The model under review builds one solid part; all positions refer to its coordinate system, in mm. Round coordinates to 2 decimals unless told otherwise and drop trailing zeros. Loops run counter-clockwise (first coordinate to the right, second up) from the corner with the lowest first, then second, coordinate; pieces in that order, holes last. Notation, with made-up numbers: (1, 28.25) -> (27, 28.25) arc R26 cw to (27, 63.25) -> close; hole circle Ø10 at (49, -3). An arc over 180 degrees is marked (long way). Return JSON: item names as keys, results as strings. Group by question number.
```python
from build123d import *

# Parameters (mm, degrees)
SKETCH1_W           = 25.4
SKETCH1_H           = 25.4
SKETCH1_W_2         = 19.05
SKETCH1_H_2         = 19.05
BOSS_EXTRUDE1_DEPTH = 266.7
CUT_EXTRUDE1_REACH  = 271.108
SKETCH3_R           = 6.35
CUT_EXTRUDE2_DEPTH  = 270.108175275


with BuildPart() as part:
    # Sketch1 → Boss-Extrude1 (new body)
    with BuildSketch(Plane.XY):
        with Locations((12.7, 12.7)):
            Rectangle(SKETCH1_W, SKETCH1_H)
        with Locations((12.7, 12.7)):
            Rectangle(SKETCH1_W_2, SKETCH1_H_2, mode=Mode.SUBTRACT)
    extrude(amount=BOSS_EXTRUDE1_DEPTH)

    # Sketch2 → Cut-Extrude1 (cut, up to next)
    with BuildSketch(Plane(origin=(0, 25.4, 0), x_dir=(1, 0, 0), z_dir=(0, 1, 0)), mode=Mode.PRIVATE) as cut_extrude1_sk1:
        Polygon((25.4, -35.938150335), (0, 0), (25.4, 0), align=None)
    cut_extrude1_tool1 = extrude(cut_extrude1_sk1.sketch, amount=-CUT_EXTRUDE1_REACH, mode=Mode.PRIVATE) & part.part
    add(cut_extrude1_tool1.solids().sort_by_distance((16.933333, 25.4, 11.979383))[0], mode=Mode.SUBTRACT)

    # Sketch3 → Cut-Extrude2 (cut, through all)
    with BuildSketch(Plane(origin=(0, 25.4, 0), x_dir=(1, 0, 0), z_dir=(0, 1, 0))):
        with Locations(Location((12.7, -241.3, 0), (0, 0, 270))):
            Circle(SKETCH3_R)
    extrude(amount=-CUT_EXTRUDE2_DEPTH, mode=Mode.SUBTRACT)


solid = part.part
```
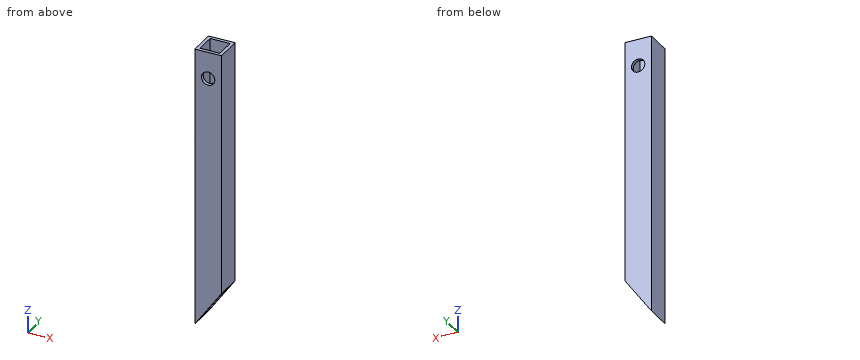
1. We need section B-B, the plane z = 241.3. Write out the cut boundary in (x, y) (3 decimals).
2. We need section D-D, the plane z = 43.5. Write out the cut boundary in (x, y) (3 decimals), then the cut area to 3 significant figures.
3. We need section C-C, the plane x = 10.25. Write out the cut boundary in (y, z) (3 decimals), then the cut area to 3 significant figures.
4. We need section A-A, the plane y = 15.5. Write out the cut boundary in (x, z) (3 decimals), then the cut area to 3 significant figures.
5. Wall thickness on line 1 (X direction, y = 19.5, z = 207.5) (3 decimals); line 2 (X direction, y = 2.3, z = 241.3): over which ranges is each line inside the solid? List them lowest first.
Check sheet entries:
{
 "1": {"outline": "(0, 0) -> (6.35, 0) -> (6.35, 3.175) -> (3.175, 3.175) -> (3.175, 22.225) -> (6.35, 22.225) -> (6.35, 25.4) -> (0, 25.4) -> close; (19.05, 0) -> (25.4, 0) -> (25.4, 25.4) -> (19.05, 25.4) -> (19.05, 22.225) -> (22.225, 22.225) -> (22.225, 3.175) -> (19.05, 3.175) -> close"},
 "2": {"outline": "(0, 0) -> (25.4, 0) -> (25.4, 25.4) -> (0, 25.4) -> close; hole (3.175, 3.175) -> (22.225, 3.175) -> (22.225, 22.225) -> (3.175, 22.225) -> close", "area": "282 mm²"},
 "3": {"outline": "(0, 14.503) -> (3.175, 14.503) -> (3.175, 235.442) -> (0, 235.442) -> close; (0, 247.158) -> (3.175, 247.158) -> (3.175, 266.7) -> (0, 266.7) -> close; (22.225, 14.503) -> (25.4, 14.503) -> (25.4, 235.442) -> (22.225, 235.442) -> close; (22.225, 247.158) -> (25.4, 247.158) -> (25.4, 266.7) -> (22.225, 266.7) -> close", "area": "1,530 mm²"},
 "4": {"outline": "(0, 0) -> (3.175, 4.492) -> (3.175, 266.7) -> (0, 266.7) -> close; (22.225, 31.446) -> (25.4, 35.938) -> (25.4, 266.7) -> (22.225, 266.7) -> close", "area": "1,580 mm²"},
 "5": {"line 1": "x = 0 to 3.175, 22.225 to 25.4", "line 2": "x = 0 to 6.35, 19.05 to 25.4"}
}
